```python
from build123d import *
from build123d.topology import SkipClean

# Parameters (mm, degrees)
SKETCH_1_R           = 255
EXTRUDE_1_DEPTH      = 1
CUT_EXTRUDE_1_DEPTH  = 361.625844886
EXTRUDE_START        = 13
EXTRUDE_3_DEPTH      = 13
CUT_EXTRUDE_6_DEPTH  = 12
SKETCH_9_R           = 50
CUT_EXTRUDE_7_DEPTH  = 14
CUT_EXTRUDE_START    = -24
CUT_EXTRUDE_8_DEPTH  = 24
CUT_EXTRUDE_9_DEPTH  = 12
SKETCH_12_R          = 3.2
CUT_EXTRUDE_10_DEPTH = 10
SKETCH_13_R          = 3.2
CUT_EXTRUDE_11_DEPTH = 10
SKETCH_14_R          = 2.25
CUT_EXTRUDE_12_DEPTH = 10
SKETCH_16_R          = 2.3
CUT_EXTRUDE_13_DEPTH = 10
SKETCH_15_R          = 2.25
CUT_EXTRUDE_14_DEPTH = 10
SKETCH_17_W          = 25
SKETCH_17_H          = 15
CUT_EXTRUDE_15_DEPTH = 4.5


with BuildPart() as part:
    # 草图1 → 拉伸1 (new body)
    with BuildSketch(Plane.XY):
        Circle(SKETCH_1_R)
    extrude(amount=EXTRUDE_1_DEPTH)

    # 草图2 → 切除-拉伸1 (cut, through all)
    with BuildSketch(Plane.XY.offset(1)):
        with BuildLine():
            Line((-74, 244.02663789), (-74, 111.900834456))
            Line((-74, 111.900834456), (-148.774990748, -17.613248654))
            Line((-148.774990748, -17.613248654), (-167.81626488, -50.593702892))
            Line((-167.81626488, -50.593702892), (-142.769914648, -93.975254038))
            Line((-142.769914648, -93.975254038), (-215.666603726, -136.0621771))
            ThreePointArc((-215.666603726, -136.0621771), (-238.942591743, 89.058620308), (-74, 244.02663789))
        make_face()
        with BuildLine():
            Line((133.908965344, 8.135462652), (248.333267613, -57.927439065))
            ThreePointArc((248.333267613, -57.927439065), (196.598323484, 162.401044341), (-10, 254.803846125))
            Line((-10, 254.803846125), (-10, 170.63))
            Line((-10, 170.63), (40.092700464, 170.63))
            Line((40.092700464, 170.63), (59.133974596, 137.649545762))
            Line((59.133974596, 137.649545762), (133.908965344, 8.135462652))
        make_face()
        with BuildLine():
            Line((-174.333267613, -186.099198825), (-59.908965344, -120.036297108))
            Line((-59.908965344, -120.036297108), (89.641016151, -120.036297108))
            Line((89.641016151, -120.036297108), (127.723564416, -120.036297108))
            Line((127.723564416, -120.036297108), (152.769914648, -76.654745962))
            Line((152.769914648, -76.654745962), (225.666603726, -118.741669025))
            ThreePointArc((225.666603726, -118.741669025), (42.344268258, -251.45966465), (-174.333267613, -186.099198825))
        make_face()
    extrude(amount=-CUT_EXTRUDE_1_DEPTH, mode=Mode.SUBTRACT)

    # 草图7 → 拉伸3 (add)
    with BuildSketch(Plane(origin=(0, 0, 0), x_dir=(-1, 0, 0), z_dir=(0, 0, -1)).offset(EXTRUDE_START)):
        with BuildLine():
            Line((-133.908965344, 8.135462652), (-248.333267613, -57.927439065))
            ThreePointArc((-248.333267613, -57.927439065), (-238.942591743, -89.058620308), (-225.666603726, -118.741669025))
            Line((-225.666603726, -118.741669025), (-152.769914648, -76.654745962))
            Line((-152.769914648, -76.654745962), (-127.723564416, -120.036297108))
            Line((-127.723564416, -120.036297108), (59.908965344, -120.036297108))
            Line((59.908965344, -120.036297108), (174.333267613, -186.099198825))
            ThreePointArc((174.333267613, -186.099198825), (196.598323484, -162.401044341), (215.666603726, -136.0621771))
            Line((215.666603726, -136.0621771), (142.769914648, -93.975254038))
            Line((142.769914648, -93.975254038), (167.81626488, -50.593702892))
            Line((167.81626488, -50.593702892), (74, 111.900834456))
            Line((74, 111.900834456), (74, 244.02663789))
            ThreePointArc((74, 244.02663789), (42.344268258, 251.45966465), (10, 254.803846125))
            Line((10, 254.803846125), (10, 170.63))
            Line((10, 170.63), (-40.092700464, 170.63))
            Line((-40.092700464, 170.63), (-133.908965344, 8.135462652))
        make_face()
    extrude(amount=-EXTRUDE_3_DEPTH)

    # 草图8 → 切除-拉伸6 (cut)
    with SkipClean():  # the faces are left unmerged after this step: merging them gives an invalid solid
        with BuildSketch(Plane(origin=(0, 0, -13), x_dir=(-1, 0, 0), z_dir=(0, 0, -1))):
            Polygon((-39.515350195, 169.63), (-133.176914536, 7.403411844), (-183.403889244, -21.595145524), (-151.903889244, -76.154745962), (-127.146214147, -119.036297108), (60.176914536, -119.036297108), (110.403889244, -148.034854476), (141.903889244, -93.475254038), (166.661564341, -50.593702892), (73, 111.632885264), (73, 169.63), (10, 169.63), align=None)
        extrude(amount=-CUT_EXTRUDE_6_DEPTH, mode=Mode.SUBTRACT)

    # 草图9 → 切除-拉伸7 (cut)
    with SkipClean():  # the faces are left unmerged after this step: merging them gives an invalid solid
        with BuildSketch(Plane(origin=(0, 0, -1), x_dir=(-1, 0, 0), z_dir=(0, 0, -1))):
            Circle(SKETCH_9_R)
        extrude(amount=-CUT_EXTRUDE_7_DEPTH, mode=Mode.SUBTRACT)

    # 草图10 → 切除-拉伸8 (cut)
    with BuildSketch(Plane.XY.offset(1).offset(CUT_EXTRUDE_START)):
        with BuildLine():
            Line((225.666603726, -118.741669025), (215.467242209, -112.853064907))
            Line((215.467242209, -112.853064907), (247.467242209, -57.427439065))
            Line((247.467242209, -57.427439065), (248.333267613, -57.927439065))
            ThreePointArc((248.333267613, -57.927439065), (238.942591743, -89.058620308), (225.666603726, -118.741669025))
        make_face()
        with BuildLine():
            Line((-74, 243.02663789), (-10, 243.02663789))
            Line((-10, 243.02663789), (-10, 254.803846125))
            ThreePointArc((-10, 254.803846125), (-42.344268258, 251.45966465), (-74, 244.02663789))
            Line((-74, 244.02663789), (-74, 243.02663789))
        make_face()
        with BuildLine():
            Line((-215.666603726, -136.0621771), (-205.467242209, -130.173572983))
            Line((-205.467242209, -130.173572983), (-173.467242209, -185.599198825))
            Line((-173.467242209, -185.599198825), (-174.333267613, -186.099198825))
            ThreePointArc((-174.333267613, -186.099198825), (-196.598323484, -162.401044341), (-215.666603726, -136.0621771))
        make_face()
    extrude(amount=CUT_EXTRUDE_8_DEPTH, mode=Mode.SUBTRACT)

    # 草图11 → 切除-拉伸9 (cut)
    with BuildSketch(Plane.XY.offset(1)):
        Polygon((-11, 170.669617313), (-73, 170.669617313), (-73, 171.63), (-73, 242.02663789), (-11, 242.02663789), (-11, 171.63), align=None)
        Polygon((153.269914648, -75.788720558), (184.269914648, -22.095145524), (246.101216805, -57.793464469), (215.101216805, -111.487039503), align=None)
        Polygon((-173.101216805, -184.233173421), (-204.101216805, -130.539598387), (-142.269914648, -94.841279442), (-111.269914648, -148.534854476), align=None)
    extrude(amount=-CUT_EXTRUDE_9_DEPTH, mode=Mode.SUBTRACT)

    # 草图12 → 切除-拉伸10 (cut)
    with BuildSketch(Plane(origin=(0, 0, -1), x_dir=(-1, 0, 0), z_dir=(0, 0, -1))):
        with Locations((-12.5, -65)):
            Circle(SKETCH_12_R)
        with Locations((12.5, -65)):
            Circle(SKETCH_12_R)
    extrude(amount=-CUT_EXTRUDE_10_DEPTH, mode=Mode.SUBTRACT)

    # 草图13 → 切除-拉伸11 (cut)
    with BuildSketch(Plane(origin=(0, 0, -1), x_dir=(-1, 0, 0), z_dir=(0, 0, -1))):
        with Locations((0, 125)):
            Circle(SKETCH_13_R)
        with Locations((108.253175473, -62.5)):
            Circle(SKETCH_13_R)
        with Locations((-108.253175473, -62.5)):
            Circle(SKETCH_13_R)
    extrude(amount=-CUT_EXTRUDE_11_DEPTH, mode=Mode.SUBTRACT)

    # 草图14 → 切除-拉伸12 (cut)
    with BuildSketch(Plane(origin=(5, -8.660254038, 0), x_dir=(-0.8660254037844386, -0.5000000000000001, 0), z_dir=(-0.5000000000000001, 0.8660254037844386, 0))):
        with Locations((208.832756681, -6.69566134)):
            Circle(SKETCH_14_R)
    extrude(amount=-CUT_EXTRUDE_12_DEPTH, mode=Mode.SUBTRACT)

    # 草图16 → 切除-拉伸13 (cut)
    with BuildSketch(Plane(origin=(-10, 0, 0), x_dir=(0, 0, -1), z_dir=(1, 0, 0))):
        with Locations(Location((6.69566134, 208.832756681, 0), (0, 0, 90))):
            Circle(SKETCH_16_R)
    extrude(amount=-CUT_EXTRUDE_13_DEPTH, mode=Mode.SUBTRACT)

    # 草图15 → 切除-拉伸14 (cut)
    with BuildSketch(Plane(origin=(5, 8.660254038, 0), x_dir=(0.8660254037844386, -0.5, 0), z_dir=(-0.5000000000000001, -0.8660254037844387, 0))):
        with Locations((208.832756681, -6.69566134)):
            Circle(SKETCH_15_R)
    extrude(amount=-CUT_EXTRUDE_14_DEPTH, mode=Mode.SUBTRACT)

    # 草图17 → 切除-拉伸15 (cut)
    with BuildSketch(Plane(origin=(0, 0, -1), x_dir=(-1, 0, 0), z_dir=(0, 0, -1))):
        with Locations((0, -107.536297108)):
            Rectangle(SKETCH_17_W, SKETCH_17_H)
    extrude(amount=-CUT_EXTRUDE_15_DEPTH, mode=Mode.SUBTRACT)


solid = part.part
```
Here's how the part is built. I have some questions about the finished solid (model axes, mm). A direction names the side the tool comes from. Coordinates: 2 decimals unless noted, no trailing zeros. Write each loop counter-clockwise with the first axis right and the second up, starting at its lowest first coordinate (ties: lowest second). Pieces come first, ordered by that corner, then holes. Notation, with made-up numbers: (14.25, 46.5) -> (52.25, 46.5) arc R27 ccw to (52.25, 66.5) -> close; hole circle Ø10 at (6, 59). An arc over 180 degrees is marked (long way). Use a Markdown table: item, result. Add a question column.
(1) I'm going to push flat-ended pins straight in: P1, Ø3.5, axis at x = -42, z = -3.5, coming from the -Y side; P2, Ø4, axis at y = 43.5, z = -0.5, coming from the -X side; P3, Ø4, axis at x = 23.5, z = -8.5, coming from the +Y side; P4, Ø6, axis at x = -108.25, y = -62.5, coming from the +Z side. Where does each tip first touch, or does it pass through?
(2) For faces 4 (the flat face through (35, -119.036, -7)), 5 (the flat face through (-157, -139, -11)), 6 (the flat face through (231.24, -85.53, -6.1)), which set-ups out of +Z, -Z, +X, -X, +Y, -Y let a thin tool reach every point of the face, with its end or its side?
(3) We'd pull the mould along X, two halves only. Please class faces 1 (the flat face through (20, -50, 1)), 2 (the flat face through (-10, 207, -5)), 3 (the flat face through (157.939, -6.893, -7.084)): +X half, -X half, draft (parallel to the pull), parting line (faces both ways), or undercut.
(4) If we section it at B-B, the plane x = 76.5: Write out the boundary of the cut face in (y, z), and give its area (3 significant figures).
(5) If we section it at A-A, the plane x = -93: Write out the boundary of the cut face in (y, z).
(6) Please list where these lines run through material, in increasing order: line 1 (X direction, y = 182.5, z = -8.25); line 2 (Y direction, x = -3.5, z = 0.25); line 3 (Y direction, x = -65.5, z = -5.25).
Outcome:
| question | item | result |
|---|---|---|
| 1 | P1 | stops at y = -120.04 |
| 1 | P2 | stops at x = -114.65 |
| 1 | P3 | stops at y = 170.63 |
| 1 | P4 | passes through |
| 2 | face 4 | -Z |
| 2 | face 5 | +Z |
| 2 | face 6 | +Z, -Z, +X, -Y |
| 3 | face 1 | draft |
| 3 | face 2 | +X half |
| 3 | face 3 | undercut |
| 4 | outline | (-120.04, -13) -> (-119.04, -13) -> (-119.04, -1) -> (105.57, -1) -> (105.57, -13) -> (107.57, -13) -> (107.57, 1) -> (-120.04, 1) -> close |
| 4 | area | 491 mm^2 |
| 5 | outline | (-139.14, -13) -> (-137.99, -13) -> (-137.99, -1) -> (76.99, -1) -> (76.99, -13) -> (78.99, -13) -> (78.99, 1) -> (-139.14, 1) -> close |
| 6 | line 1 | x = -74 to -73, -11 to -10 |
| 6 | line 2 | y = -120.04 to -115.04, -100.04 to -49.88, 49.88 to 170.63 |
| 6 | line 3 | y = -123.26 to -122.11, 169.63 to 170.67, 242.03 to 243.03 |
